Could you check a few things on this model? Use its own coordinates, in mm. A direction names the side the tool comes from. Round coordinates to 2 decimals unless told otherwise and drop trailing zeros. Order: outer loops, then holes, each group sorted by start corner. A loop starts at its lowest first (then second) coordinate and runs counter-clockwise, first axis right, second up. Notation, with made-up numbers: (69, -6.75) -> (103, -6.75) arc R13 ccw to (103, 6.25) -> close; hole circle Ø7 at (1, 70). An arc over 180 degrees is marked (long way). Put each result on its own line as item: value. Start each with the question number.
from build123d import *

# Parameters (mm, degrees)
SKIZZE1_W                          = 37.873435046
SKIZZE1_H                          = 37.873435047
AUFSATZ_LINEAR_AUSTRAGEN1_DEPTH    = 20
SKIZZE2_R                          = 10.575
SCHNITT_LINEAR_AUSTRAGEN1_DEPTH    = 4
SKIZZE3_W                          = 12
SKIZZE3_H                          = 12
SCHNITT_LINEAR_AUSTRAGEN3_DEPTH    = 7.5
VERRUNDUNG1_R                      = 8
KREISMUSTER1_COUNT                 = 4
SKIZZE4_R                          = 8.775
SCHNITT_LINEAR_AUSTRAGEN4_DEPTH    = 0.5
K_RPER_VERSCHIEBEN_KOPIEREN1_ANGLE = 90
SCHNITT_LINEAR_AUSTRAGEN5_DEPTH    = 21
SCHNITT_LINEAR_START               = -6
SKIZZE6_R                          = 1.45
SCHNITT_LINEAR_AUSTRAGEN6_DEPTH    = 16
KREISMUSTER2_COUNT                 = 4
SKIZZE7_W                          = 35.652729611
SKIZZE7_H                          = 9.273531579
SCHNITT_LINEAR_AUSTRAGEN8_DEPTH    = 45.41348481
SKIZZE8_W                          = 12.4
SKIZZE8_H                          = 12.2
SCHNITT_LINEAR_AUSTRAGEN9_DEPTH    = 7.5
KREISMUSTER11_COUNT                = 4
FASE1_SIZE                         = 0.5
VERRUNDUNG2_R                      = 0.5


with BuildPart() as part:
    # Skizze1 → Aufsatz-Linear austragen1 (new body)
    with BuildSketch(Plane(origin=(0, 0, 0), x_dir=(1, 0, 0), z_dir=(0, 1, 0))):
        with Locations((6, 12.936717524)):
            Rectangle(SKIZZE1_W, SKIZZE1_H)
    extrude(amount=AUFSATZ_LINEAR_AUSTRAGEN1_DEPTH)

    # Skizze2 → Schnitt-Linear austragen1 (cut)
    with BuildSketch(Plane.XZ):
        with Locations((6, -12.936717523)):
            Circle(SKIZZE2_R)
    extrude(amount=-SCHNITT_LINEAR_AUSTRAGEN1_DEPTH, mode=Mode.SUBTRACT)

    # Skizze3 → Schnitt-Linear austragen3 (cut)
    with BuildSketch(Plane.XY.offset(6)):
        with Locations((6, 9.2)):
            Rectangle(SKIZZE3_W, SKIZZE3_H)
    schnitt_linear_austragen3 = extrude(amount=-SCHNITT_LINEAR_AUSTRAGEN3_DEPTH, mode=Mode.SUBTRACT)

    # Verrundung1
    verrundung1_edges = [part.edges().sort_by_distance(p)[0] for p in [
        (24.936717523, 10, -31.873435047),
        (24.936717523, 10, 6),
        (-12.936717523, 10, 6),
        (-12.936717523, 10, -31.873435047),
    ]]
    fillet(verrundung1_edges, radius=VERRUNDUNG1_R)

    # Kreismuster1: Schnitt-Linear austragen3 ×4 about axis
    kreismuster1_axis = Axis((6, 0, -12.936717523), (0, 1, 0))
    for i in range(1, KREISMUSTER1_COUNT):
        add(schnitt_linear_austragen3.rotate(kreismuster1_axis, i * 360 / KREISMUSTER1_COUNT), mode=Mode.SUBTRACT)

    # Skizze4 → Schnitt-Linear austragen4 (cut)
    with BuildSketch(Plane.XZ.offset(-4)):
        with Locations((6, -12.936717523)):
            Circle(SKIZZE4_R)
    extrude(amount=-SCHNITT_LINEAR_AUSTRAGEN4_DEPTH, mode=Mode.SUBTRACT)


with BuildPart() as part_1:
    # Körper-Verschieben/Kopieren1: moved
    add(part.part.rotate(Axis((0, 10, -12.936717523), (-1, 0, 0)), K_RPER_VERSCHIEBEN_KOPIEREN1_ANGLE))

    # Skizze5 → Schnitt-Linear austragen5 (cut, through all)
    with BuildSketch(Plane.XY.offset(-2.936717523)):
        Polygon((0, 28.936717523), (-12.936717523, 16), (-12.936717523, 28.936717523), align=None)
        Polygon((24.936717523, 16), (24.936717523, 28.936717523), (12, 28.936717523), align=None)
        Polygon((12, -8.936717523), (24.936717523, 4), (24.936717523, -8.936717523), align=None)
        Polygon((-12.936717523, -8.936717523), (0, -8.936717523), (-12.936717523, 4), align=None)
    extrude(amount=-SCHNITT_LINEAR_AUSTRAGEN5_DEPTH, mode=Mode.SUBTRACT)

    # Skizze6 → Schnitt-Linear austragen6 (cut)
    with BuildSketch(Plane(origin=(-14.468358762, 14.468358762, 0), x_dir=(0.707106781, 0.707106781, 0), z_dir=(-0.707106781, 0.707106781, 0)).offset(SCHNITT_LINEAR_START)):
        with Locations((11.284238529, 12.936717523)):
            Circle(SKIZZE6_R)
    schnitt_linear_austragen6 = extrude(amount=SCHNITT_LINEAR_AUSTRAGEN6_DEPTH, mode=Mode.SUBTRACT)

    # Kreismuster2: Schnitt-Linear austragen6 ×4 about axis
    kreismuster2_axis = Axis((6, 10, 0), (0, 0, 1))
    for i in range(1, KREISMUSTER2_COUNT):
        add(schnitt_linear_austragen6.rotate(kreismuster2_axis, i * 360 / KREISMUSTER2_COUNT), mode=Mode.SUBTRACT)

    # Skizze7 → Schnitt-Linear austragen8 (cut, through all)
    with BuildSketch(Plane(origin=(20.468358762, 20.468358762, 0), x_dir=(0.707106781, -0.707106781, 0), z_dir=(0.707106781, 0.707106781, 0))):
        with Locations((-3.021869868, 23.873483313)):
            Rectangle(SKIZZE7_W, SKIZZE7_H)
    extrude(amount=-SCHNITT_LINEAR_AUSTRAGEN8_DEPTH, mode=Mode.SUBTRACT)

    # Skizze8 → Schnitt-Linear austragen9 (cut)
    with BuildSketch(Plane.ZY.offset(12.936717523)):
        with Locations((-12.036717523, 10)):
            Rectangle(SKIZZE8_W, SKIZZE8_H)
    schnitt_linear_austragen9 = extrude(amount=-SCHNITT_LINEAR_AUSTRAGEN9_DEPTH, mode=Mode.SUBTRACT)

    # Kreismuster11: Schnitt-Linear austragen9 ×4 about axis
    kreismuster11_axis = Axis((6, 10, 0), (0, 0, 1))
    for i in range(1, KREISMUSTER11_COUNT):
        add(schnitt_linear_austragen9.rotate(kreismuster11_axis, i * 360 / KREISMUSTER11_COUNT), mode=Mode.SUBTRACT)

    # Fase1
    fase1_edges = [part_1.edges().sort_by_distance(p)[0] for p in [
        (-12.936717523, 10, -2.936717523),
        (6, -8.936717523, -2.936717523),
        (24.936717523, 10, -2.936717523),
        (6, 28.936717523, -2.936717523),
        (-6.468358762, -2.468358762, -2.936717523),
        (18.468358762, -2.468358762, -2.936717523),
        (18.468358762, 22.468358762, -2.936717523),
        (-4.575, 10, -2.936717523),
        (-6.468358762, 22.468358762, -2.936717523),
        (-7.51450201, 21.422215513, -12.936717523),
        (-5.422215513, -3.51450201, -12.936717523),
        (19.51450201, -1.422215513, -12.936717523),
        (17.422215513, 23.51450201, -12.936717523),
        (-6.468358762, 22.468358762, -19.236717523),
        (18.468358762, 22.468358762, -19.236717523),
        (18.468358762, -2.468358762, -19.236717523),
        (24.936717523, 10, -19.236717523),
        (6, 28.936717523, -19.236717523),
        (-12.936717523, 10, -19.236717523),
        (-6.468358762, -2.468358762, -19.236717523),
        (6, -8.936717523, -19.236717523),
    ]]
    chamfer(fase1_edges, length=FASE1_SIZE)

    # Verrundung2
    verrundung2_edges = [part_1.edges().sort_by_distance(p)[0] for p in [
        (-12.836717523, 16.1, -12.036717523),
        (-12.836717523, 3.9, -12.036717523),
        (-0.1, 28.836717523, -12.036717523),
        (12.1, 28.836717523, -12.036717523),
        (24.836717523, 16.1, -12.036717523),
        (-0.1, -8.836717523, -12.036717523),
        (24.836717523, 3.9, -12.036717523),
        (12.1, -8.836717523, -12.036717523),
    ]]
    fillet(verrundung2_edges, radius=VERRUNDUNG2_R)


solid = part_1.part
1. Which directions (+Z, -Z, +X, -X, +Y, -Y) give clear straight access to the entire face, cutting with the end or side of a thin tool? Please do faces 5 (the face through (-5.437, 10, -12)), 6 (the face through (12.416, -8.095, -11.95)), 7 (the face through (-0.1, 25, -12)), 8 (the face through (21, 10, -5.837)).
2. I need wall thicknesses on L1, parallel to Z at x = -6.5, y = 12; L2, parallel to Y at x = 6, z = -7.3 (3 decimals); L3, parallel to Y at x = 6, z = -5.05 (3 decimals). Which ranges of each line are inside material? Lowest first, please.
3. If we section it at B-B, the plane x = 6: Please give me the cut outline in (y, z) (3 decimals).
4. If we section it at C-C, the plane y = 25.5: Please give me the cut outline in (x, z), then the cut area to 3 significant figures.
5. For pin 1 Ø3.5 at (y, z) = (12.5, -13) entering from -X; pin 2 Ø4 at (y, z) = (17.5, -14.5) entering from -X; pin 3 Ø2 at (x, y) = (8, 16.5) entering from +Z, each with a flat end and sliding along its axis, tell me the tip position at first contact or that it passes through.
6. If we section it at A-A, the plane y = 10: Please give me the cut outline in (x, z) (3 decimals).
7. Thinking about a two-plate mould opening in X: for faces 1 (the face through (24.095, 16.416, -12.124)), 2 (the face through (-0.1, -5, -12)), 3 (the face through (-9, 3.9, -12)), 4 (the face through (-6.2, -2.4, -3.2)), which applies, +X half, -X half, draft (parallel to the pull), parting line (faces both ways), or undercut?
8. If we section it at D-D, the plane z = -16.25: Please give me the cut outline in (x, y), then the cut area to 3 significant figures.
Results below:
1. face 5: -X
1. face 6: -Y
1. face 7: +Y
1. face 8: +X
2. L1: -19.24 to -18.24, -5.84 to -2.94
2. L2: -1.437 to 1.225, 18.775 to 21.437
2. L3: -8.937 to -0.575, 20.575 to 28.937
3. outline: (-8.937, -18.737) -> (-8.437, -19.237) -> (28.437, -19.237) -> (28.937, -18.737) -> (28.937, -18.237) -> (21.437, -18.237) -> (21.437, -5.837) -> (28.937, -5.837) -> (28.937, -3.437) -> (28.437, -2.937) -> (21.075, -2.937) -> (20.575, -3.437) -> (20.575, -6.937) -> (18.775, -6.937) -> (18.775, -7.437) -> (1.225, -7.437) -> (1.225, -6.937) -> (-0.575, -6.937) -> (-0.575, -3.437) -> (-1.075, -2.937) -> (-8.437, -2.937) -> (-8.937, -3.437) -> (-8.937, -5.837) -> (-1.437, -5.837) -> (-1.437, -18.237) -> (-8.937, -18.237) -> close
4. outline: (-3.44, -18.74) -> (-2.73, -19.24) -> (14.73, -19.24) -> (15.44, -18.74) -> (15.44, -3.44) -> (14.73, -2.94) -> (-2.73, -2.94) -> (-3.44, -3.44) -> close; hole (-0.1, -18.24) -> (12.1, -18.24) -> (12.1, -5.84) -> (-0.1, -5.84) -> close
4. area: 156 mm2
5. pin 1: x = -5.44
5. pin 2: x = -12.13
5. pin 3: z = -7.44
6. outline: (-12.937, -18.737) -> (-12.437, -19.237) -> (24.437, -19.237) -> (24.937, -18.737) -> (24.937, -18.237) -> (17.437, -18.237) -> (17.437, -5.837) -> (24.937, -5.837) -> (24.937, -3.437) -> (24.437, -2.937) -> (17.075, -2.937) -> (16.575, -3.437) -> (16.575, -6.937) -> (14.775, -6.937) -> (14.775, -7.437) -> (-2.775, -7.437) -> (-2.775, -6.937) -> (-4.575, -6.937) -> (-4.575, -3.437) -> (-5.075, -2.937) -> (-12.437, -2.937) -> (-12.937, -3.437) -> (-12.937, -5.837) -> (-5.437, -5.837) -> (-5.437, -18.237) -> (-12.937, -18.237) -> close
7. face 1: +X half
7. face 2: undercut
7. face 3: draft
7. face 4: -X half
8. outline: (-11.98, 3.05) -> (-0.95, -7.98) arc R0.5 ccw to (-0.1, -7.63) -> (-0.1, -1.44) -> (12.1, -1.44) -> (12.1, -7.63) arc R0.5 ccw to (12.95, -7.98) -> (23.98, 3.05) arc R0.5 ccw to (23.63, 3.9) -> (17.44, 3.9) -> (17.44, 16.1) -> (23.63, 16.1) arc R0.5 ccw to (23.98, 16.95) -> (12.95, 27.98) arc R0.5 ccw to (12.1, 27.63) -> (12.1, 21.44) -> (-0.1, 21.44) -> (-0.1, 27.63) arc R0.5 ccw to (-0.95, 27.98) -> (-11.98, 16.95) arc R0.5 ccw to (-11.63, 16.1) -> (-5.44, 16.1) -> (-5.44, 3.9) -> (-11.63, 3.9) arc R0.5 ccw to start
8. area: 731 mm2
